The model under review builds one solid part; all positions refer to its coordinate system, in mm. Face numbers are marked on the shaded views. Give positions to 0.01 mm unless a question says otherwise; leave off trailing zeros. Loops run counter-clockwise (first coordinate to the right, second up) from the corner with the lowest first, then second, coordinate; pieces in that order, holes last. Notation, with made-up numbers: M 33,56.25 L 51,56.25 A26 cw 51,73.25 Z; hole C 16,-6.5 d6. An arc over 180 degrees is marked long. Return JSON: item names as keys, results as strings. Group by question number.
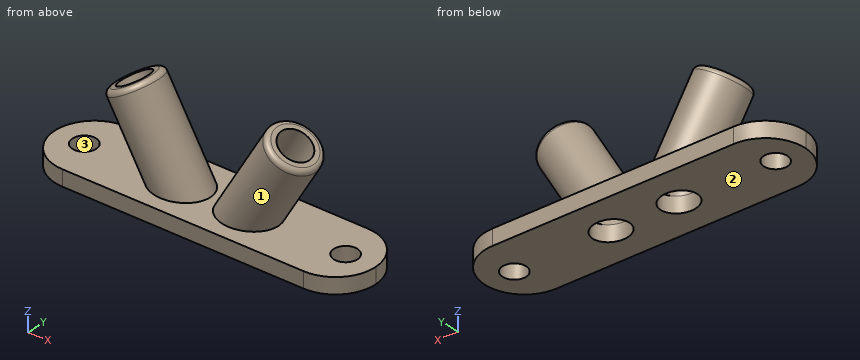
```python
from build123d import *

# Parameters (mm, degrees)
F0_W      = 40
F0_H      = 10
F0_R      = 1.5
F1_DEPTH  = 2
F7_R      = 3.2
F7_R_2    = 2
F9_R      = 3.2
F9_R_2    = 2
F11_R     = 4.99999
F12_DEPTH = 2.001
F13_DEPTH = 2.0010001
F14_R     = 0.6


# Not quite as in the source:
# - a fillet or chamfer is up to 0.001 mm smaller than in the source, because OpenCascade refuses the exact size


with BuildPart() as f1:
    # F0 (on Top) → F1 (new body)
    with BuildSketch(Plane.XY):
        Rectangle(F0_W, F0_H)
        with Locations((-16.25, 0)):
            Circle(F0_R, mode=Mode.SUBTRACT)
        with Locations((16.25, 0)):
            Circle(F0_R, mode=Mode.SUBTRACT)
    extrude(amount=F1_DEPTH)

    # F7 (on line) → F8 (join, up to the next surface of F1)
    with BuildSketch(Plane(origin=(7.6961524227, 0, 13.3301270189), x_dir=(0.8660254038, 0, -0.5), z_dir=(-0.5, 0, -0.8660254038))):
        with Locations((2.6602540378, 0)):
            Circle(F7_R)
        with Locations((2.6602540378, 0)):
            Circle(F7_R_2, mode=Mode.SUBTRACT)
    extrude(until=Until.NEXT)

    # F9 (on line) → F10 (join, up to the next surface of F1)
    with BuildSketch(Plane(origin=(-7.6961524227, 0, 13.3301270189), x_dir=(0.8660254038, 0, 0.5), z_dir=(0.5, 0, -0.8660254038))):
        with Locations((-2.6602540378, 0)):
            Circle(F9_R)
        with Locations((-2.6602540378, 0)):
            Circle(F9_R_2, mode=Mode.SUBTRACT)
    extrude(until=Until.NEXT)

    # F11 (radius 5 in the source; OpenCascade refuses exactly that, so slightly less here)
    f11_edges = [f1.edges().sort_by_distance(p)[0] for p in [
        (-20, -5, 1),
        (20, -5, 1),
        (20, 5, 1),
        (-20, 5, 1),
    ]]
    fillet(f11_edges, radius=F11_R)

    # F12 (cut, through all): a face of the model
    f12_faces = [f1.faces().sort_by_distance(p)[0] for p in [
        (-4.2264973081, 0, 2),
    ]]
    extrude(f12_faces, amount=-F12_DEPTH, mode=Mode.SUBTRACT)

    # F13 (cut, through all): a face of the model
    f13_faces = [f1.faces().sort_by_distance(p)[0] for p in [
        (4.2264973081, 0, 2),
    ]]
    extrude(f13_faces, amount=-F13_DEPTH, mode=Mode.SUBTRACT)

    # F14
    f14_edges = [f1.edges().sort_by_distance(p)[0] for p in [
        (-12.771281, 0, 10.4),
        (7.228719, 0, 13.6),
    ]]
    fillet(f14_edges, radius=F14_R)


solid = f1.part
```
(1) For probe 1 along X at (y, z) = (-0.5, 1.75); probe 2 along X at (y, z) = (-0.25, 5); probe 3 along X at (y, z) = (1.25, 9), list the stretches that pass through material, from the lowest coordinate up.
(2) Add section A-A (x = -16). Write out the cut boundary in (y, z), and give its area (3 significant figures).
(3) Add section C-C (x = 16.25). Write out the cut boundary in (y, z), and give its area (3 significant figures).
(4) Add section B-B (z = 8). Count the separate pieces of the cut face and the enclosed holes in it, and give its area (3 significant figures).
(5) For pin 1 (1.5 mm diameter, centred on x = 13, y = 2, fed in from +Z); pin 2 (1.5 mm diameter, centred on y = 0, z = 8.5, fed in from -X); pin 3 (6 mm diameter, centred on x = 7.5, y = 3.5, fed in from +Z); pin 4 (2.5 mm diameter, centred on x = 16.25, y = 0, fed in from -Z), all flat-tipped, find the tip position at first contact; note any pin that passes through.
(6) Mouldability with a two-part tool opening along Z and no side actions: class the marked faces 1, 2 and 3 as released by +Z, released by -Z, zero draft, split by the parting line, or undercut.
Verdict:
{
 "1": {"probe 1": "x = -19.97 to -17.66, -14.84 to -6.46, -1.99 to 1.99, 6.46 to 14.84, 17.66 to 19.97", "probe 2": "x = -9.64 to -8.25, -3.67 to -2.27, 2.27 to 3.67, 8.25 to 9.64", "probe 3": "x = -11.67 to -10.07, -6.47 to -4.87, 4.87 to 6.47, 10.07 to 11.67"},
 "2": {"outline": "M -4.9,0 L -1.48,0 L -1.48,2 L -4.9,2 Z; M 1.48,0 L 4.9,0 L 4.9,2 L 1.48,2 Z", "area": "13.7 mm²"},
 "3": {"outline": "M -4.84,0 L -1.5,0 L -1.5,2 L -4.84,2 Z; M 1.5,0 L 4.84,0 L 4.84,2 L 1.5,2 Z", "area": "13.4 mm²"},
 "4": {"separate pieces": "2", "enclosed holes": "2", "area": "45.3 mm²"},
 "5": {"pin 1": "stops at z = 2", "pin 2": "stops at x = -12.11", "pin 3": "stops at z = 13.36", "pin 4": "passes through"},
 "6": {"face 1": "undercut", "face 2": "released by -Z", "face 3": "zero draft"}
}
